Work out the finished part from the listing and answer in its coordinate system (mm). Round coordinates to 2 decimals unless told otherwise and drop trailing zeros. Write item = value, one per line. Start each with the question number.
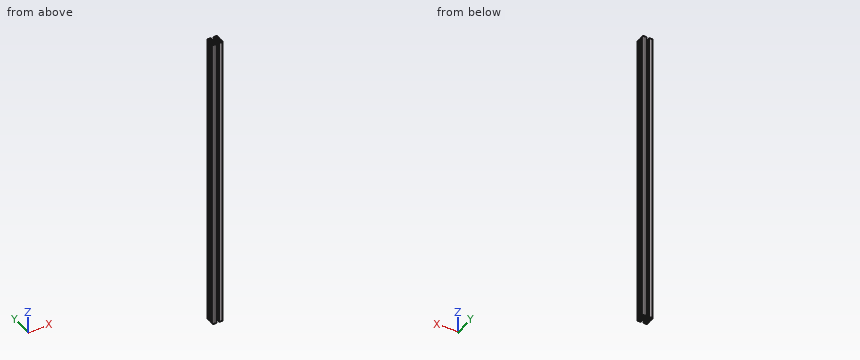
```python
from build123d import *

# Parameters (mm, degrees)
F1_DEPTH = 914.4


# Not quite as in the source:
# - ends of sketch curves that miss each other by under 0.0002 mm in the source are joined


with BuildPart() as f1:
    # F0 (on Top) → F1 (new body)
    with BuildSketch(Plane.XY):
        with BuildLine():
            Line((-10.053123, -8.25), (-12.8, -8.25))
            Line((-12.8, -8.25), (-12.800036, -4.05))
            Line((-12.800036, -4.05), (-14.5, -4.05))
            Line((-14.5, -4.05), (-14.5, -4.55))
            Line((-14.5, -4.55), (-15, -4.55))
            Line((-15, -4.55), (-15, -13))
            ThreePointArc((-15, -13), (-14.4142135624, -14.4142135624), (-13, -15))
            Line((-13, -15), (-4.55, -15))
            Line((-4.55, -15), (-4.55, -14.5))
            Line((-4.55, -14.5), (-4.05, -14.5))
            Line((-4.05, -14.5), (-4.05, -12.800036))
            Line((-4.05, -12.800036), (-8.25, -12.8))
            Line((-8.25, -12.8), (-8.25, -10.053123))
            Line((-8.25, -10.053123), (-4.196877, -6))
            Line((-4.196877, -6), (4.196877, -6))
            Line((4.196877, -6), (8.25, -10.053123))
            Line((8.25, -10.053123), (8.25, -12.8))
            Line((8.25, -12.8), (4.05, -12.800036))
            Line((4.05, -12.800036), (4.05, -14.5))
            Line((4.05, -14.5), (4.55, -14.5))
            Line((4.55, -14.5), (4.55, -15))
            Line((4.55, -15), (13, -15))
            ThreePointArc((13, -15), (14.4142135624, -14.4142135624), (15, -13))
            Line((15, -13), (15, -4.55))
            Line((15, -4.55), (14.5, -4.55))
            Line((14.5, -4.55), (14.5, -4.05))
            Line((14.5, -4.05), (12.800036, -4.05))
            Line((12.800036, -4.05), (12.8, -8.25))
            Line((12.8, -8.25), (10.053123, -8.25))
            Line((10.053123, -8.25), (6, -4.196877))
            Line((6, -4.196877), (6, 4.196877))
            Line((6, 4.196877), (10.053123, 8.25))
            Line((10.053123, 8.25), (12.8, 8.25))
            Line((12.8, 8.25), (12.800036, 4.05))
            Line((12.800036, 4.05), (14.5, 4.05))
            Line((14.5, 4.05), (14.5, 4.55))
            Line((14.5, 4.55), (15, 4.55))
            Line((15, 4.55), (15, 13))
            ThreePointArc((15, 13), (14.4142135624, 14.4142135624), (13, 15))
            Line((13, 15), (4.55, 15))
            Line((4.55, 15), (4.55, 14.5))
            Line((4.55, 14.5), (4.05, 14.5))
            Line((4.05, 14.5), (4.05, 12.800036))
            Line((4.05, 12.800036), (8.25, 12.8))
            Line((8.25, 12.8), (8.25, 10.053123))
            Line((8.25, 10.053123), (4.196877, 6))
            Line((4.196877, 6), (-4.196877, 6))
            Line((-4.196877, 6), (-8.25, 10.053123))
            Line((-8.25, 10.053123), (-8.25, 12.8))
            Line((-8.25, 12.8), (-4.05, 12.800036))
            Line((-4.05, 12.800036), (-4.05, 14.5))
            Line((-4.05, 14.5), (-4.55, 14.5))
            Line((-4.55, 14.5), (-4.55, 15))
            Line((-4.55, 15), (-13, 15))
            ThreePointArc((-13, 15), (-14.4142135624, 14.4142135624), (-15, 13))
            Line((-15, 13), (-15, 4.55))
            Line((-15, 4.55), (-14.5, 4.55))
            Line((-14.5, 4.55), (-14.5, 4.05))
            Line((-14.5, 4.05), (-12.800036, 4.05))
            Line((-12.800036, 4.05), (-12.8, 8.25))
            Line((-12.8, 8.25), (-10.053123, 8.25))
            Line((-10.053123, 8.25), (-6, 4.196877))
            Line((-6, 4.196877), (-6, -4.196877))
            Line((-6, -4.196877), (-10.053123, -8.25))
        make_face()
        with BuildLine():
            Line((-9.7, -13.85), (-12.85, -13.85))
            ThreePointArc((-12.85, -13.85), (-13.5571067812, -13.5571067812), (-13.85, -12.85))
            Line((-13.85, -12.85), (-13.85, -9.7))
            Line((-13.85, -9.7), (-9.7, -9.7))
            Line((-9.7, -9.7), (-9.7, -13.85))
        make_face(mode=Mode.SUBTRACT)
        with BuildLine():
            Line((12.85, -13.85), (9.7, -13.85))
            Line((9.7, -13.85), (9.7, -9.7))
            Line((9.7, -9.7), (13.85, -9.7))
            Line((13.85, -9.7), (13.85, -12.85))
            ThreePointArc((13.85, -12.85), (13.5571067812, -13.5571067812), (12.85, -13.85))
        make_face(mode=Mode.SUBTRACT)
        with BuildLine():
            Line((-9.7, 9.7), (-13.85, 9.7))
            Line((-13.85, 9.7), (-13.85, 12.85))
            ThreePointArc((-13.85, 12.85), (-13.5571067812, 13.5571067812), (-12.85, 13.85))
            Line((-12.85, 13.85), (-9.7, 13.85))
            Line((-9.7, 13.85), (-9.7, 9.7))
        make_face(mode=Mode.SUBTRACT)
        with BuildLine():
            Line((3.272394, -1.616767), (4.590523, -3.187652))
            Line((4.590523, -3.187652), (3.187652, -4.590523))
            Line((3.187652, -4.590523), (1.616767, -3.272394))
            ThreePointArc((1.616767, -3.272394), (0, -3.65), (-1.6167671199, -3.2723942427))
            Line((-1.6167671199, -3.2723942427), (-3.187652, -4.590523))
            Line((-3.187652, -4.590523), (-4.590523, -3.187652))
            Line((-4.590523, -3.187652), (-3.272394, -1.616767))
            ThreePointArc((-3.272394, -1.616767), (-3.65, 0), (-3.2723942427, 1.6167671199))
            Line((-3.2723942427, 1.6167671199), (-4.590523, 3.187652))
            Line((-4.590523, 3.187652), (-3.187652, 4.590523))
            Line((-3.187652, 4.590523), (-1.616767, 3.272394))
            ThreePointArc((-1.616767, 3.272394), (0, 3.65), (1.6167671199, 3.2723942427))
            Line((1.6167671199, 3.2723942427), (3.187652, 4.590523))
            Line((3.187652, 4.590523), (4.590523, 3.187652))
            Line((4.590523, 3.187652), (3.272394, 1.616767))
            ThreePointArc((3.272394, 1.616767), (3.65, 0), (3.272394, -1.616767))
        make_face(mode=Mode.SUBTRACT)
        with BuildLine():
            Line((13.85, 9.7), (9.7, 9.7))
            Line((9.7, 9.7), (9.7, 13.85))
            Line((9.7, 13.85), (12.85, 13.85))
            ThreePointArc((12.85, 13.85), (13.5571067812, 13.5571067812), (13.85, 12.85))
            Line((13.85, 12.85), (13.85, 9.7))
        make_face(mode=Mode.SUBTRACT)
    extrude(amount=F1_DEPTH)


solid = f1.part
```
Item 1: Flat-ended cylindrical pins translate along their axes: pin 1 (4 mm diameter, centred on x = 1.5, z = 108, fed in from +Y); pin 2 (0.6 mm diameter, centred on x = -4, z = 611.5, fed in from +Y); pin 3 (4 mm diameter, centred on y = 0.5, z = 333.5, fed in from -X). Find the tip coordinate at first contact, or state that the pin passes through.
Item 2: Section A-A (z = 205) is taken. Count the separate pieces of the cut face and the enclosed holes in it, then the cut area to 3 significant figures.
Item 3: Find the intervals of material crossed by line 1 along Y through (x, z) = (-12.75, 520.5); line 2 along X through (y, z) = (13, 312.5), in increasing order. Write a range as [from, to].
Worked answers:
q1.pin_1 = 6
q1.pin_2 = 14.5
q1.pin_3 = -6
q2.separate_pieces = 1
q2.enclosed_holes = 5
q2.area = 314 mm2
q3.line_1 = [-15, -13.85], [-9.7, -8.25], [8.25, 9.7], [13.85, 15]
q3.line_2 = [-15, -13.84], [-9.7, -4.05], [4.05, 9.7], [13.84, 15]
